from build123d import *

# Parameters (mm, degrees)
SKETCH_W      = 13
SKETCH_H      = 10
PAD_DEPTH     = 1.6
SKETCH001_R   = 1.5
SKETCH001_W   = 0.65
SKETCH001_H   = 0.65
POCKET_DEPTH  = 5
SKETCH002_W   = 2.6
SKETCH002_H   = 2.6
PAD001_DEPTH  = 0.03
SKETCH003_W   = 2.1
SKETCH003_H   = 2.1
PAD002_DEPTH  = 0.9
FILLET_R      = 0.3
FILLET001_R   = 0.05
FILLET002_R   = 0.2
SKETCH004_W   = 1.1
SKETCH004_H   = 2
SKETCH004_W_2 = 1.5
SKETCH004_H_2 = 0.9
SKETCH004_H_3 = 0.75
SKETCH004_H_4 = 2.9
SKETCH004_W_3 = 3.2
SKETCH004_H_5 = 1.4
SKETCH004_W_4 = 0.8
SKETCH004_H_6 = 1.6
PAD003_DEPTH  = 1


with BuildPart() as part:
    # Sketch (on XY_Plane of Origin) → Pad (new body)
    with BuildSketch(Plane.XY):
        with Locations((6.5, 5)):
            Rectangle(SKETCH_W, SKETCH_H)
    extrude(amount=PAD_DEPTH)

    # Sketch001 (on XY_Plane of Origin) → Pocket (cut)
    with BuildSketch(Plane.XY):
        with Locations((10.4, 7.6)):
            Circle(SKETCH001_R)
        with Locations((1.4, 8.6)):
            Rectangle(SKETCH001_W, SKETCH001_H)
        with Locations((1.4, 6.2)):
            Rectangle(SKETCH001_W, SKETCH001_H)
        with Locations((1.4, 3.8)):
            Rectangle(SKETCH001_W, SKETCH001_H)
        with Locations((1.4, 1.4)):
            Rectangle(SKETCH001_W, SKETCH001_H)
    extrude(amount=POCKET_DEPTH, mode=Mode.SUBTRACT)

    # Sketch002 (on Face5 of Pocket) → Pad001 (join)
    with BuildSketch(Plane.XY.offset(1.6)):
        with Locations((10.6, 2.7)):
            Rectangle(SKETCH002_W, SKETCH002_H)
    extrude(amount=PAD001_DEPTH)

    # Sketch003 (on Face28 of Pad001) → Pad002 (join)
    with BuildSketch(Plane.XY.offset(1.63)):
        with Locations((10.6, 2.7)):
            Rectangle(SKETCH003_W, SKETCH003_H)
    extrude(amount=PAD002_DEPTH)

    # Fillet
    fillet_edges = [part.edges().sort_by_distance(p)[0] for p in [
        (9.55, 1.65, 2.08),
        (9.55, 3.75, 2.08),
        (11.65, 1.65, 2.08),
        (11.65, 3.75, 2.08),
    ]]
    fillet(fillet_edges, radius=FILLET_R)

    # Fillet001
    fillet001_edges = [part.edges().sort_by_distance(p)[0] for p in [
        (9.637868, 1.737868, 1.63),
    ]]
    fillet(fillet001_edges, radius=FILLET001_R)

    # Fillet002
    fillet002_edges = [part.edges().sort_by_distance(p)[0] for p in [
        (10.6, 1.65, 2.53),
    ]]
    fillet(fillet002_edges, radius=FILLET002_R)

    # Sketch004 (on Face53 of Fillet002) → Pad003 (join)
    with BuildSketch(Plane(origin=(0, 0, 0), x_dir=(1, 0, 0), z_dir=(0, 0, -1))):
        with Locations((5.65, -2.1)):
            Rectangle(SKETCH004_W, SKETCH004_H)
        with Locations((8.7, -1.35)):
            Rectangle(SKETCH004_W_2, SKETCH004_H_2)
        with Locations((8.7, -2.95)):
            Rectangle(SKETCH004_W_2, SKETCH004_H_2)
        with Locations((8.7, -4.425)):
            Rectangle(SKETCH004_W_2, SKETCH004_H_3)
        with Locations((5.85, -7.65)):
            Rectangle(SKETCH004_W, SKETCH004_H_4)
        with Locations((4.8, -4.8)):
            Rectangle(SKETCH004_W_3, SKETCH004_H_5)
        with Locations((3.3, -8)):
            Rectangle(SKETCH004_W_4, SKETCH004_H_6)
    extrude(amount=PAD003_DEPTH)


solid = part.part
Check sheet for the modelled part. Datum: model origin and axes. Units: mm. A direction names the side the tool comes from. Give positions to 0.01 mm unless a question says otherwise; leave off trailing zeros. Write each loop counter-clockwise with the first axis right and the second up, starting at its lowest first coordinate (ties: lowest second). Pieces come first, ordered by that corner, then holes. Notation, with made-up numbers: (45, 80.5) -> (101, 80.5) arc R20 cw to (101, 108.5) -> close; hole circle Ø1 at (73, 4.25). An arc over 180 degrees is marked (long way). Use one line per item in the form item = value. Start each with the question number.
1. Section check A-A (y = 1.25). Record the cut outline in (x, z) (3 decimals), and give its area (3 significant figures).
2. Section check D-D (y = 7.6). Record the cut outline in (x, z), and give its area (3 significant figures).
3. Access from +Z, -Z, +X, -X, +Y, -Y to the whole of each face (thin tool, end or side, straight path). Record for faces 4 (the flat face through (6.2, 2.1, -0.5)), 5 (the flat face through (8.7, 4.8, -0.5)), 6 (the flat face through (5.8, 9.1, -0.5)).
4. Section check B-B (z = 0.35). Record the cut outline in (x, y) (3 decimals), and give its area (3 significant figures).
5. Go/stop test with a flat-tipped pin: P1, Ø0.8, axis at x = 5.5, z = -0.5, coming from the -Y side. Record where the tip stops, or that it passes through.
6. Mould release check, pull along X, two halves, no side actions. Record for faces 1 (the flat face through (0, 5, 1)), 2 (the flat face through (5.3, 7.7, -0.5)), 3 (the flat face through (6, 2, -1)): pulls with the +X half, pulls with the -X half, needs draft (parallel to the pull), parting line crosses it, or undercut.
7. Thickness scan on line 1 along X through (y, z) = (7.6, 0.55); line 2 along Y through (x, z) = (10.4, 0.9); line 3 along X through (y, z) = (6, 0.05) (3 decimals). Record the ranges inside material, lowest first. Write a range as from..to.
Conclusion:
q1.outline = (0, 0) -> (1.075, 0) -> (1.075, 1.6) -> (0, 1.6) -> close; (1.725, 0) -> (5.1, 0) -> (5.1, -1) -> (6.2, -1) -> (6.2, 0) -> (7.95, 0) -> (7.95, -1) -> (9.45, -1) -> (9.45, 0) -> (13, 0) -> (13, 1.6) -> (1.725, 1.6) -> close
q1.area = 22.4 mm²
q2.outline = (0, 0) -> (2.9, 0) -> (2.9, -1) -> (3.7, -1) -> (3.7, 0) -> (5.3, 0) -> (5.3, -1) -> (6.4, -1) -> (6.4, 0) -> (8.9, 0) -> (8.9, 1.6) -> (0, 1.6) -> close; (11.9, 0) -> (13, 0) -> (13, 1.6) -> (11.9, 1.6) -> close
q2.area = 17.9 mm²
q3.face_4 = -Z, -Y
q3.face_5 = -Z, +X, +Y
q3.face_6 = -Z, +X, -X, +Y
q4.outline = (0, 0) -> (13, 0) -> (13, 10) -> (0, 10) -> close; hole (1.075, 1.075) -> (1.725, 1.075) -> (1.725, 1.725) -> (1.075, 1.725) -> close; hole (1.075, 3.475) -> (1.725, 3.475) -> (1.725, 4.125) -> (1.075, 4.125) -> close; hole (1.075, 5.875) -> (1.725, 5.875) -> (1.725, 6.525) -> (1.075, 6.525) -> close; hole (1.075, 8.275) -> (1.725, 8.275) -> (1.725, 8.925) -> (1.075, 8.925) -> close; hole circle Ø3 at (10.4, 7.6)
q4.area = 121 mm²
q5.P1 = 1.1
q6.face_1 = pulls with the -X half
q6.face_2 = undercut
q6.face_3 = needs draft
q7.line_1 = 0..8.9, 11.9..13
q7.line_2 = 0..6.1, 9.1..10
q7.line_3 = 0..1.075, 1.725..13
